from build123d import *

# Parameters (mm, degrees)
SKETCH_1_W      = 20
SKETCH_1_H      = 15
EXTRUDE_1_DEPTH = 3
FILLET_1_R      = 2
FILLET_3_SIZE   = 2


with BuildPart() as part:
    # 草图1 → 凸台-拉伸1 (new, symmetric)
    with BuildSketch(Plane.XY):
        Rectangle(SKETCH_1_W, SKETCH_1_H)
    extrude(amount=EXTRUDE_1_DEPTH, both=True)

    # 圆角1
    fillet_1_edges = [part.edges().sort_by_distance(p)[0] for p in [
        (0, 7.5, 3),
    ]]
    fillet(fillet_1_edges, radius=FILLET_1_R)

    # 圆角3
    # a fillet whose section is not a circle: 2 mm, written as the material it takes off along each edge
    with BuildSketch(Plane(origin=(10, 12.5, -3), x_dir=(-1, 0, 0), z_dir=(0, -1, 0))) as fillet_3_piece_1:
        with BuildLine():
            Bezier((FILLET_3_SIZE, 0), (0, 0), (0, -FILLET_3_SIZE), weights=[1, 0.141421356, 1])
            Line((0, -FILLET_3_SIZE), (0, 0))
            Line((0, 0), (FILLET_3_SIZE, 0))
        make_face()
    extrude(amount=25, mode=Mode.SUBTRACT)


solid = part.part
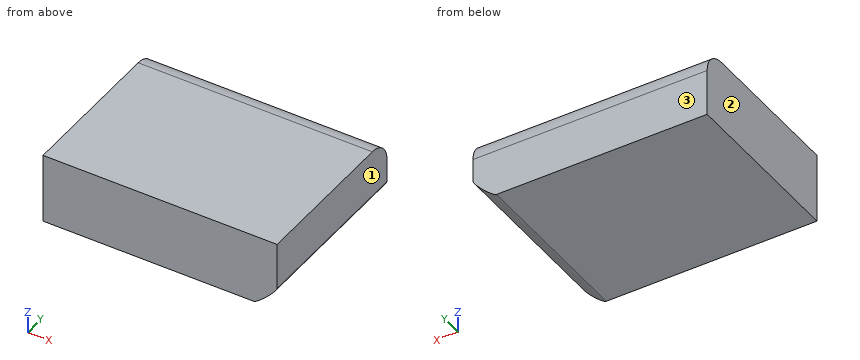
Build history of the part. All positions in model axes, mm. Face numbers are marked on the shaded views. Give positions to 0.01 mm unless a question says otherwise; leave off trailing zeros. Loops run counter-clockwise (first coordinate to the right, second up) from the corner with the lowest first, then second, coordinate; pieces in that order, holes last. Notation, with made-up numbers: (61, 44) - (75, 44) arc R34 cw to (75, 82) - close; hole circle Ø1 at (31.5, 60). An arc over 180 degrees is marked (long way). Write item = value, one per line. Start each with the question number.
1) Pull direction X, two halves, no side cores. Call the marked faces 1, 2 and 3: +X half, -X half, draft (parallel to the pull), parting line (faces both ways), or undercut.
2) Probe probe 1 along Y at (x, z) = (9.25, 2.25); probe 2 along Y at (x, z) = (-8.25, 1.5); probe 3 along X at (y, z) = (-3, -1.75). List the from-to ranges inside material, lowest first. Write a range as from..to.
3) Band-saw the part on A-A on z = 2.75. Give the cut face in (x, y), plus the area to 3 significant figures.
Final values:
q1.face_1 = +X half
q1.face_2 = -X half
q1.face_3 = draft
q2.probe_1 = -7.5..7.06
q2.probe_2 = -7.5..7.44
q2.probe_3 = -10..9.48
q3.outline = (-10, -7.5) - (10, -7.5) - (10, 6.47) - (-10, 6.47) - close
q3.area = 279 mm²
